```python
from build123d import *

# Parameters (mm, degrees)
SKETCH2_R                = 1
BOSS_EXTRUDE1_DEPTH      = 1
BOSS_EXTRUDE2_DEPTH      = 3.5
BOSS_EXTRUDE2_DEPTH_BACK = 1.25
SKETCH2_3_R              = 1


with BuildPart() as part:
    # Sketch2 → Boss-Extrude1 (new body)
    with BuildSketch(Plane.YZ):
        with BuildLine():
            ThreePointArc((-2.205882353, 3.140971298), (-7.25, 0), (-2.205882353, -3.140971298))
            ThreePointArc((-2.205882353, -3.140971298), (0, -2.628073151), (2.205882353, -3.140971298))
            ThreePointArc((2.205882353, -3.140971298), (7.25, 0), (2.205882353, 3.140971298))
            ThreePointArc((2.205882353, 3.140971298), (0, 2.628073151), (-2.205882353, 3.140971298))
        make_face()
        with Locations(Location((-3.75, 0, 0), (0, 0, 270))):
            Circle(SKETCH2_R, mode=Mode.SUBTRACT)
        with Locations(Location((3.75, 0, 0), (0, 0, 270))):
            Circle(SKETCH2_R, mode=Mode.SUBTRACT)
    extrude(amount=-BOSS_EXTRUDE1_DEPTH)

    # Sketch2_3 → Boss-Extrude2 (add, two sides: drawn at the far end of the back side and taken through both)
    with BuildSketch(Plane.YZ.offset(-BOSS_EXTRUDE2_DEPTH_BACK)):
        with Locations(Location((-3.75, 0, 0), (0, 0, 270))):
            Circle(SKETCH2_3_R)
        with Locations(Location((3.75, 0, 0), (0, 0, 270))):
            Circle(SKETCH2_3_R)
    extrude(amount=BOSS_EXTRUDE2_DEPTH + BOSS_EXTRUDE2_DEPTH_BACK)

    # Mirror1: part across plane


with BuildPart() as part_1:
    add(part.part)
    add(part.part.mirror(Plane(origin=(3.5, 0, 0), x_dir=(0, 0, 1), z_dir=(1, 0, 0))))


solid = part_1.part
```
The model under review builds one solid part; all positions refer to its coordinate system, in mm. A direction names the side the tool comes from. Coordinates: 2 decimals unless noted, no trailing zeros. Order: outer loops, then holes, each group sorted by start corner. A loop starts at its lowest first (then second) coordinate and runs counter-clockwise, first axis right, second up. Notation, with made-up numbers: (29.25, 9) -> (36.25, 9) arc R8 cw to (36.25, 20) -> close; hole circle Ø11 at (28.25, -27.5). An arc over 180 degrees is marked (long way). Answer in a Markdown table with one row per item. Add a question column.
Item 1: To check wall thickness, follow probe 1 along X at (y, z) = (-6.5, -1.75); probe 2 along Y at (x, z) = (6.5, -0.25); probe 3 along Y at (x, z) = (1.25, -0.5). State the ranges of each line that lie inside material, in increasing order.
Item 2: We need section D-D on z = 1.5. Write out the cut boundary in (x, y).
Item 3: Mouldability with a two-part tool opening along Y and no side actions: class faces 4 (the cylindrical face through (7.49, 7.25, -0.1)), 5 (the flat face through (-1.25, 4, 0)) as +Y half, -Y half, draft (parallel to the pull), parting line (faces both ways), or undercut.
Item 4: Clearance check with flat-ended pins moving along their axes: pin 1 (1.5 mm diameter, centred on x = 7, z = -2, fed in from +Y); pin 2 (1.5 mm diameter, centred on x = 6, y = -3.5, fed in from +Z); pin 3 (4 mm diameter, centred on y = -2, z = 1.5, fed in from +X); pin 4 (3 mm diameter, centred on y = -0.5, z = 0, fed in from +X). State where each tip first meets the part, or that it passes through.
Item 5: We need section B-B on x = 4.5. Write out the cut boundary in (y, z), plus the area to 3 significant figures.
Item 6: We need section A-A on y = 0. Write out the cut boundary in (x, z), plus the area to 3 significant figures.
Item 7: Machinability: for faces 1 (the flat face through (7, 0, 0)), 2 (the flat face through (-1, 0, 0)), 3 (the cylindrical face through (-0.49, 0.03, 2.63)), which of the approach directions +Z, -Z, +X, -X, +Y, -Y give a long, thin tool a straight path to every point of the face, cutting with its end or side? Answer none if there is none.
Final values:
| question | item | result |
|---|---|---|
| 1 | probe 1 | x = -1 to 0, 7 to 8 |
| 1 | probe 2 | y = -4.72 to -2.78, 2.78 to 4.72 |
| 1 | probe 3 | y = -4.62 to -2.88, 2.88 to 4.62 |
| 2 | outline | (-1, -6.91) -> (0, -6.91) -> (0, 6.91) -> (-1, 6.91) -> close; (7, -6.91) -> (8, -6.91) -> (8, 6.91) -> (7, 6.91) -> close |
| 3 | face 4 | undercut |
| 3 | face 5 | draft |
| 4 | pin 1 | stops at y = 7.02 |
| 4 | pin 2 | stops at z = 1 |
| 4 | pin 3 | stops at x = 8.25 |
| 4 | pin 4 | stops at x = 8 |
| 5 | outline | circle Ø2 at (-3.75, 0); circle Ø2 at (3.75, 0) |
| 5 | area | 6.28 mm2 |
| 6 | outline | (-1, -2.63) -> (0, -2.63) -> (0, 2.63) -> (-1, 2.63) -> close; (7, -2.63) -> (8, -2.63) -> (8, 2.63) -> (7, 2.63) -> close |
| 6 | area | 10.5 mm2 |
| 7 | face 1 | none |
| 7 | face 2 | -X |
| 7 | face 3 | +Z, +X, -X |
